Autodesk Inventor part; units mm, degrees
ref_plane "YZ Plane" through (0, 0, 0) normal (1, 0, 0) x (0, 1, 0)
ref_plane "XZ Plane" through (0, 0, 0) normal (0, 1, 0) x (-1, 0, 0)
ref_plane "XY Plane" through (0, 0, 0) normal (0, 0, 1) x (1, 0, 0)
sketch "Sketch1" plane through (0, 0, 0) normal (0, 0, 1) x (1, 0, 0)
  line L0 (23.778, 63) -> (8.751, 62.999)
  line L1 (8.7511, 59.9974) -> (8.751, 62.999)
  line L2 (-8.7484, 59.9988) -> (8.7511, 59.9974)
  line L3 (-8.7482, 62.8637) -> (-8.7484, 59.9988)
  line L4 (-8.7482, 62.8637) -> (-23.7781, 63.0002)
  circle A0 centre (11.7, 47.6838) radius 8.25
  circle A1 centre (-11.7, 47.6838) radius 8.25
  circle A2 centre (0.0002, 40.7838) radius 2.95
  circle A3 centre (19.375, 39.6228) radius 1.5875
  circle A4 centre (-19.375, 55.7448) radius 1.5875
  line L5 (10.98, 11.2972) -> (-10.98, 11.2972)
  arc A5 (13.638, 8.6392) -> (10.98, 11.2972) centre (10.98, 8.6392) ccw
  arc A6 (-10.98, 11.2972) -> (-13.638, 8.6392) centre (-10.98, 8.6392) ccw
  line L6 (-0.0001, 27) -> (-7.6501, 27) construction
  line L7 (-7.6501, 27) -> (-0.0001, 27) construction
  line L8 (-0.0001, 34) -> (-0.0001, 27) construction
  line L9 (10, 0) -> (20, 0)
  line L10 (-20, 0) -> (-10, 0)
  line L11 (-5, 0) -> (5, 0) construction
  line L12 (20, 0) -> (20, 3.0003)
  line L13 (20, 3.0003) -> (23.778, 3)
  line L14 (10, 0) -> (10, 3.0012)
  line L15 (-10, 3.0012) -> (-10, 0)
  line L16 (-20, 0) -> (-20, 3)
  line L17 (-20, 3) -> (-23.7781, 3)
  line L18 (13.638, 8.6392) -> (13.638, 5.0012)
  line L19 (-13.638, 8.6392) -> (-13.638, 5.0012)
  line L20 (11.638, 3.0012) -> (10, 3.0012)
  line L21 (-10, 3.0012) -> (-11.638, 3.0012)
  arc A7 (11.638, 3.0012) -> (13.638, 5.0012) centre (11.638, 5.0012) ccw
  arc A8 (-13.638, 5.0012) -> (-11.638, 3.0012) centre (-11.638, 5.0012) ccw
  line L22 (23.778, 28) -> (26.778, 28)
  line L23 (26.778, 28) -> (26.778, 38)
  line L24 (26.778, 38) -> (23.778, 38)
  line L25 (23.778, 48) -> (26.778, 48)
  line L26 (26.778, 48) -> (26.778, 58)
  line L27 (26.778, 58) -> (23.778, 58)
  line L28 (23.778, 8) -> (26.778, 8)
  line L29 (26.778, 8) -> (26.778, 18)
  line L30 (26.778, 18) -> (23.778, 18)
  line L31 (23.778, 28) -> (26.778, 28)
  line L32 (26.778, 28) -> (26.778, 38)
  line L33 (26.778, 38) -> (23.778, 38)
  line L34 (23.778, 48) -> (23.778, 38)
  line L35 (23.778, 28) -> (23.778, 18)
  line L36 (23.778, 8) -> (23.778, 3)
  line L37 (-23.7781, 28) -> (-26.7781, 28)
  line L38 (-26.7781, 28) -> (-26.7781, 38)
  line L39 (-26.7781, 38) -> (-23.7781, 38)
  line L40 (-26.7781, 48) -> (-26.7781, 58)
  line L41 (-26.7781, 58) -> (-23.7781, 58)
  line L42 (-23.7781, 48) -> (-26.7781, 48)
  line L43 (-26.7781, 8) -> (-26.7781, 18)
  line L44 (-26.7781, 18) -> (-23.7781, 18)
  line L45 (-23.7781, 8) -> (-26.7781, 8)
  line L46 (-26.7781, 28) -> (-26.7781, 38)
  line L47 (-26.7781, 38) -> (-23.7781, 38)
  line L48 (-23.7781, 28) -> (-26.7781, 28)
  line L49 (-23.7781, 48) -> (-23.7781, 38)
  line L50 (-23.7781, 28) -> (-23.7781, 18)
  circle A9 centre (0.0002, 54.5838) radius 2.95
  line L51 (0.0002, 50) -> (0.0002, 45) construction
  line L52 (10, 47.6838) -> (6, 47.6838) construction
  circle A10 centre (19.375, 55.7448) radius 1.5875
  circle A11 centre (-19.375, 39.6228) radius 1.5875
  line L53 (-23.7781, 3) -> (-23.7781, 8)
  line L54 (23.778, 63) -> (23.778, 58)
  line L55 (-23.7781, 63.0002) -> (-23.7781, 58)
  line L56 (23.778, 63) -> (23.778, 62.5)
  line L57 (23.778, 63) -> (22.778, 63)
  line L58 (23.778, 63) -> (24.778, 63) construction
  line L59 (22.778, 63) -> (22.778, 58)
  line L60 (22.778, 58) -> (23.778, 58)
  line L61 (23.778, 48) -> (22.778, 48)
  line L62 (22.778, 48) -> (22.778, 38)
  line L63 (22.778, 38) -> (23.778, 38)
  line L64 (23.778, 28) -> (22.778, 28)
  line L65 (22.778, 28) -> (22.778, 18)
  line L66 (22.778, 18) -> (23.778, 18)
  line L67 (23.778, 8) -> (22.778, 8)
  line L68 (22.778, 8) -> (22.7776, 3.0001)
  line L69 (-23.7781, 63.0002) -> (-23.7781, 62.5002)
  line L70 (-23.7781, 63.0002) -> (-22.7781, 62.9911)
  line L71 (-22.7781, 62.9911) -> (-22.8235, 57.9913)
  line L72 (-22.8235, 57.9913) -> (-23.7781, 58)
  line L73 (-23.7781, 48) -> (-22.9143, 47.9922)
  line L74 (-22.9143, 47.9922) -> (-23.0051, 37.9926)
  line L75 (-23.0051, 37.9926) -> (-24.0051, 38)
  line L76 (-23.7781, 28) -> (-22.7781, 28)
  line L77 (-22.7781, 28) -> (-22.7781, 18)
  line L78 (-22.7781, 18) -> (-23.7781, 18)
  line L79 (-23.7781, 8) -> (-22.7781, 8)
  line L80 (-23.7781, 8) -> (-22.7781, 8) construction
  line L81 (-22.7781, 8) -> (-22.7781, 3)
  point P0 (0, 0)
  point P1 (0, 1.5)
  point P2 (15, 0)
  point P3 (15, 1.5)
  point P4 (-15, 0)
  point P5 (-15, 1.5)
  point P6 (0, 0)
  point P7 (0, 1.5)
  point P8 (13.638, 3.0012)
  point P9 (-23.7781, 23)
  dimension "d4" = 15
  dimension "d7" = 15
  dimension "d11" = 2
  dimension "d12" = 3
  dimension "d16" = 20
  dimension "d19" = 20
  dimension "d46" = 7.675
  dimension "d47" = 7.675
  dimension "d50" = 0.5
  dimension "d51" = 1
  dimension "d52" = 180
  dimension "d53" = 10
  dimension "d54" = 10
  dimension "d55" = 90
  dimension "d56" = 1
  dimension "d57" = 0.5
  dimension "d58" = 1
  dimension "d59" = 5
  dimension "d60" = 10
  dimension "d61" = 1
  dimension "d62" = 1
  dimension "d63" = 1
  dimension "d64" = 0
  dimension "d67" = 8.061
  dimension "d68" = 8.061
  dimension "d69" = 1
  dimension "d70" = 1
extrude "Extrusion1" add sketch "Sketch1" along normal blind 3
extrude "Extrusion2" cut sketch "Sketch1" along normal up to next contours L54 L60 L59 L0 | L34 L63 L62 L61 | L71 L72 L55 L4 | L35 L66 L65 L64 | L73 L74 L75 L49 | L36 L13 L68 L67 | L76 L77 L78 L50 | L79 L81 L17 L53
sketch "Sketch2" plane through (0, 0, 0) normal (0, 0, -1) x (-1, 0, 0)
  line L0 (-22.778, 8) -> (-26.778, 8)
  line L1 (-26.778, 58) -> (-24.778, 58)
  line L2 (-24.778, 58) -> (-24.778, 8)
  line L3 (-24.778, 8) -> (-26.778, 8)
  line L4 (-26.778, 8) -> (-26.778, 58)
  line L5 (26.7781, 8) -> (22.7781, 8)
  line L6 (26.7781, 58) -> (24.7781, 58)
  line L7 (24.7781, 58) -> (24.7781, 8)
  line L8 (24.7781, 8) -> (26.7781, 8)
  line L9 (26.7781, 8) -> (26.7781, 58)
  point P0 (0, 0)
extrude "Extrusion3" cut sketch "Sketch2" against normal through all
equation "\"d56\" = d51"
equation "\"d58\" = d51"
equation "\"d61\" = d51"
equation "\"d62\" = d51"
equation "\"d63\" = d51"
equation "\"d68\" = d67"
equation "\"d69\" = d51"
equation "\"d70\" = d51"
properties part number "srf depan"
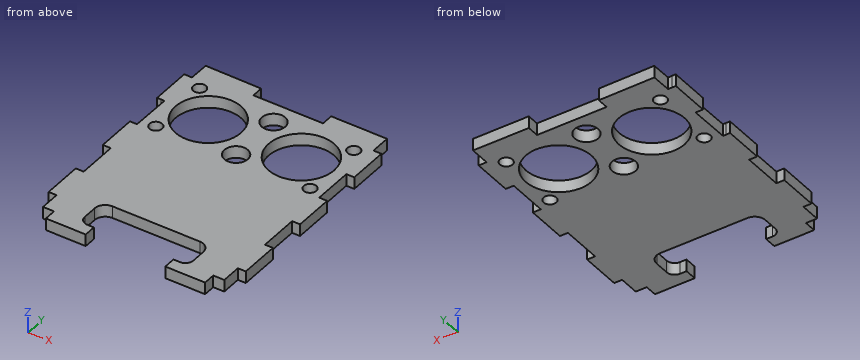
The listing builds one solid part. Answer for the finished solid, in the listing's coordinates (mm). Coordinates: 2 decimals unless noted, no trailing zeros. Loops run counter-clockwise (first coordinate to the right, second up) from the corner with the lowest first, then second, coordinate; pieces in that order, holes last. Notation, with made-up numbers: (61, 71) -> (100, 71) arc R18 cw to (100, 91) -> close; hole circle Ø11 at (41, 62). An arc over 180 degrees is marked (long way). Return JSON: item names as keys, results as strings. Group by question number.
(1) A cutting plane is placed at C-C on x = 2. Write down the section's boundary in (y, z), and give its area (3 significant figures).
(2) A cutting plane is placed at B-B on x = 7. Write down the section's boundary in (y, z), and give its area (3 significant figures).
(3) A cutting plane is placed at A-A on x = 19. Write down the section's boundary in (y, z), and give its area (3 significant figures).
(4) A cutting plane is placed at D-D on z = 1.35. Count the separate pieces of the cut face and the enclosed holes in it, and give its area (3 significant figures).
(5) Given pin 1 Ø1 at (x, z) = (24, 2) entering from -Y; pin 2 Ø0.9 at (x, z) = (5, 2) entering from -Y; pin 3 Ø1.3 at (x, z) = (-10.5, 2) entering from +Y, each flat-ended and moving along its own axis, determine where each tip first touches the part or whether it passes through.
(6) Find the intervals of material crossed by probe 1 along X at (y, z) = (54, 0.7); probe 2 along X at (y, z) = (41, 0.75); probe 3 along Y at (x, z) = (1, 2.75), in increasing order. Write a range as from..to.
The answers:
{
 "1": {"outline": "(11.3, 0) -> (38.62, 0) -> (38.62, 3) -> (11.3, 3) -> close; (42.95, 0) -> (52.42, 0) -> (52.42, 3) -> (42.95, 3) -> close; (56.75, 0) -> (60, 0) -> (60, 3) -> (56.75, 3) -> close", "area": "120 mm^2"},
 "2": {"outline": "(11.3, 0) -> (40.9, 0) -> (40.9, 3) -> (11.3, 3) -> close; (54.46, 0) -> (60, 0) -> (60, 3) -> (54.46, 3) -> close", "area": "105 mm^2"},
 "3": {"outline": "(0, 0) -> (38.08, 0) -> (38.08, 3) -> (0, 3) -> close; (41.17, 0) -> (43.84, 0) -> (43.84, 3) -> (41.17, 3) -> close; (51.53, 0) -> (54.2, 0) -> (54.2, 3) -> (51.53, 3) -> close; (57.29, 0) -> (63, 0) -> (63, 3) -> (57.29, 3) -> close", "area": "147 mm^2"},
 "4": {"separate pieces": "1", "enclosed holes": "8", "area": "2,130 mm^2"},
 "5": {"pin 1": "stops at y = 8", "pin 2": "stops at y = 11.3", "pin 3": "stops at y = 62.89"},
 "6": {"probe 1": "x = -24.78..-17.01, -6.39..-2.89, 2.89..6.39, 17.01..24.78", "probe 2": "x = -22.98..-20.16, -18.59..-16.54, -6.86..-2.94, 2.94..6.86, 16.54..18.59, 20.16..22.78", "probe 3": "y = 11.3..38.01, 43.56..51.81, 57.36..60"}
}
